from build123d import *

# Parameters (mm, degrees)
F0_W     = 233
F0_H     = 430
F1_DEPTH = 2
F2_W     = 85
F2_H     = 30
F2_W_2   = 61.5
F2_H_2   = 33
F2_W_3   = 2
F2_H_3   = 25
F2_R     = 2
F3_DEPTH = 2.001


with BuildPart() as f1:
    # F0 (on Top) → F1 (new body)
    with BuildSketch(Plane.XY):
        Rectangle(F0_W, F0_H)
    extrude(amount=F1_DEPTH)

    # F2 (on face) → F3 (cut, through all)
    with BuildSketch(Plane.XY.offset(2)):
        with Locations((-74, 200)):
            Rectangle(F2_W, F2_H)
        with Locations((74, 200)):
            Rectangle(F2_W, F2_H)
        with Locations((-35.75, -183.25)):
            Rectangle(F2_W_2, F2_H_2)
        with Locations((35.75, -183.25)):
            Rectangle(F2_W_2, F2_H_2)
        with Locations((-115.5, -132.5)):
            Rectangle(F2_W_3, F2_H_3)
        with Locations((115.5, -132.5)):
            Rectangle(F2_W_3, F2_H_3)
        with Locations((-111, 132.77711)):
            Circle(F2_R)
        with Locations((111, 132.77711)):
            Circle(F2_R)
        with Locations((-111, 63.28708)):
            Circle(F2_R)
        with Locations((111, 63.28708)):
            Circle(F2_R)
        with Locations((-111, -43.205046)):
            Circle(F2_R)
        with Locations((111, -43.205046)):
            Circle(F2_R)
        with Locations((111, -200)):
            Circle(F2_R)
        with Locations((-111, -200)):
            Circle(F2_R)
        with Locations((0, 29.134061)):
            Circle(F2_R)
    extrude(amount=-F3_DEPTH, mode=Mode.SUBTRACT)


solid = f1.part
Check sheet for the modelled part. Datum: model origin and axes. Units: mm. Give positions to 0.01 mm unless a question says otherwise; leave off trailing zeros. Write each loop counter-clockwise with the first axis right and the second up, starting at its lowest first coordinate (ties: lowest second). Pieces come first, ordered by that corner, then holes. Notation, with made-up numbers: (78.5, 72.25) -> (117.5, 72.25) arc R26 ccw to (117.5, 98.25) -> close; hole circle Ø7 at (82.5, 77). An arc over 180 degrees is marked (long way). One line per item, written item: value. Start each with the question number.
Item 1: Gauge pin test, flat ends, axial feed: pin 1 (1 mm diameter, centred on y = -137, z = 0, fed in from -X); pin 2 (0.6 mm diameter, centred on y = 199, z = 1, fed in from -X). Record the tip position at first contact, or that the pin passes through.
Item 2: Section check B-B on z = 1.3. State how many separate pieces and enclosed holes the cut face has, then the cut area to 3 significant figures.
Item 3: Material ranges on probe 1 along Y at (x, z) = (111, 1.05); probe 2 along Y at (x, z) = (-47.5, 1.35); probe 3 along Y at (x, z) = (96, 1.55), recorded low to high. Write a range as from..to.
Item 4: Section check A-A on x = 53.5. Record the cut outline in (y, z).
Item 5: Section check C-C on y = -129. Record the cut outline in (x, z).
Results list:
1. pin 1: x = -114.5
1. pin 2: x = -31.5
2. separate pieces: 1
2. enclosed holes: 11
2. area: 90,800 mm²
3. probe 1: -215..-202, -198..-45.21, -41.21..61.29, 65.29..130.78, 134.78..185
3. probe 2: -215..-199.75, -166.75..185
3. probe 3: -215..185
4. outline: (-215, 0) -> (-199.75, 0) -> (-199.75, 2) -> (-215, 2) -> close; (-166.75, 0) -> (185, 0) -> (185, 2) -> (-166.75, 2) -> close
5. outline: (-114.5, 0) -> (114.5, 0) -> (114.5, 2) -> (-114.5, 2) -> close
